Here's how the part is built. I have some questions about the finished solid (model axes, mm). A direction names the side the tool comes from. Round coordinates to 2 decimals unless told otherwise and drop trailing zeros. Loops run counter-clockwise (first coordinate to the right, second up) from the corner with the lowest first, then second, coordinate; pieces in that order, holes last. Notation, with made-up numbers: M -9.75,60 L 39.25,60 A17 ccw 39.25,90 Z; hole C 51.25,20.25 d4. An arc over 180 degrees is marked long. Use a Markdown table: item, result.
from build123d import *

# Parameters (mm, degrees)
SKETCH1_W                 = 101.6
SKETCH1_H                 = 48.26
BOSS_EXTRUDE1_DEPTH       = 38.1
SHELL1_T                  = -7.62
SKETCH4_W                 = 22.86
SKETCH4_H                 = 10.16
CUT_EXTRUDE1_DEPTH        = 38.1
SKETCH5_W                 = 33.02
SKETCH5_H                 = 7.62
CUT_EXTRUDE2_DEPTH        = 80.757617818
F_8_32_TAPPED_HOLE1_D     = 3.4544
F_8_32_TAPPED_HOLE1_DEPTH = 12.065
F_8_32_TAPPED_HOLE1_TIP   = 1.037806461


with BuildPart() as part:
    # Sketch1 → Boss-Extrude1 (new body)
    with BuildSketch(Plane(origin=(0, 0, 0), x_dir=(1, 0, 0), z_dir=(0, 1, 0))):
        Rectangle(SKETCH1_W, SKETCH1_H)
    extrude(amount=BOSS_EXTRUDE1_DEPTH)

    # Shell1
    shell1_openings = [part.faces().sort_by_distance(p)[0] for p in [
        (0, 38.1, 0),
    ]]
    offset(amount=SHELL1_T, openings=shell1_openings, kind=Kind.INTERSECTION)

    # Sketch4 → Cut-Extrude1 (cut)
    with BuildSketch(Plane.ZY.offset(50.8)):
        with Locations((0, 19.685)):
            Rectangle(SKETCH4_W, SKETCH4_H)
    extrude(amount=-CUT_EXTRUDE1_DEPTH, mode=Mode.SUBTRACT)

    # Sketch5 → Cut-Extrude2 (cut, through all)
    with BuildSketch(Plane(origin=(0, 0, -24.13), x_dir=(-1, 0, 0), z_dir=(0, 0, -1))):
        with Locations((-21.234297506, 19.685)):
            Rectangle(SKETCH5_W, SKETCH5_H)
    extrude(amount=-CUT_EXTRUDE2_DEPTH, mode=Mode.SUBTRACT)

    # #8-32 Tapped Hole1
    with Locations(Plane(origin=(0, 38.1, 0), x_dir=(1, 0, 0), z_dir=(0, 1, 0))):
        with Locations((46.99, -20.32), (26.67, 0), (46.99, 20.32), (6.35, -20.32), (6.35, 20.32)):
            Hole(F_8_32_TAPPED_HOLE1_D / 2, depth=F_8_32_TAPPED_HOLE1_DEPTH)
            with Locations((0, 0, -(F_8_32_TAPPED_HOLE1_DEPTH + F_8_32_TAPPED_HOLE1_TIP / 2))):  # 118° drill point
                Cone(0, F_8_32_TAPPED_HOLE1_D / 2, F_8_32_TAPPED_HOLE1_TIP, mode=Mode.SUBTRACT)


solid = part.part
1. Which directions (+Z, -Z, +X, -X, +Y, -Y) give clear straight access to the entire face, cutting with the end or side of a thin tool? Please do faces 1 (the face through (-47, 20, 11.43)), 2 (the face through (50.8, 19, 0)), 3 (the face through (-50.8, 10, 0)), 4 (the face through (5.421, 31.983, -21.776)), 5 (the face through (37.744, 20, 20)).
Answer sheet:
| item | result |
|---|---|
| face 1 | -X |
| face 2 | +Z, -Z, +X, +Y, -Y |
| face 3 | +Z, -Z, -X, +Y, -Y |
| face 4 | +Y |
| face 5 | +Z, -Z |
2. Imagine slicing it at D-D, the plane y = 34. Write out the boundary of the cut face in (x, z), then the cut area to 3 significant figures.
Answer sheet:
| item | result |
|---|---|
| outline | M -50.8,-24.13 L 50.8,-24.13 L 50.8,24.13 L -50.8,24.13 Z; hole M -43.18,-16.51 L 43.18,-16.51 L 43.18,16.51 L -43.18,16.51 Z; hole C 6.35,-20.32 d3.45; hole C 6.35,20.32 d3.45; hole C 46.99,-20.32 d3.45; hole C 46.99,20.32 d3.45 |
| area | 2,010 mm2 |
3. Imagine slicing it at A-A, the plane x = 9.5. Write out the boundary of the cut face in (y, z) (3 decimals), then the cut area to 3 significant figures.
Answer sheet:
| item | result |
|---|---|
| outline | M 0,-24.13 L 15.875,-24.13 L 15.875,-16.51 L 7.62,-16.51 L 7.62,16.51 L 15.875,16.51 L 15.875,24.13 L 0,24.13 Z; M 23.495,-24.13 L 38.1,-24.13 L 38.1,-16.51 L 23.495,-16.51 Z; M 23.495,16.51 L 38.1,16.51 L 38.1,24.13 L 23.495,24.13 Z |
| area | 716 mm2 |
4. Imagine slicing it at B-B, the plane y = 19.5. Write out the boundary of the cut face in (x, z).
Answer sheet:
| item | result |
|---|---|
| outline | M -50.8,-24.13 L 4.72,-24.13 L 4.72,-16.51 L -43.18,-16.51 L -43.18,-11.43 L -50.8,-11.43 Z; M -50.8,11.43 L -43.18,11.43 L -43.18,16.51 L 4.72,16.51 L 4.72,24.13 L -50.8,24.13 Z; M 37.74,-24.13 L 50.8,-24.13 L 50.8,24.13 L 37.74,24.13 L 37.74,16.51 L 43.18,16.51 L 43.18,-16.51 L 37.74,-16.51 Z |
5. We'd pull the mould along Y, two halves only. Please class faces 6 (the face through (-1, 19, 24.13)), 7 (the face through (47.151, 25.177, -20.573)), 8 (the face through (-47, 14.605, 0)): +Y half, -Y half, draft (parallel to the pull), parting line (faces both ways), or undercut.
Answer sheet:
| item | result |
|---|---|
| face 6 | draft |
| face 7 | +Y half |
| face 8 | undercut |
6. For pin 1 Ø1.5 at (x, z) = (-17.5, -4) entering from +Y, with a flat end and sliding along its axis, tell me the tip position at first contact or that it passes through.
Answer sheet:
| item | result |
|---|---|
| pin 1 | y = 7.62 |
7. Imagine slicing it at C-C, the plane z = 5. Write out the boundary of the cut face in (x, y) (3 decimals).
Answer sheet:
| item | result |
|---|---|
| outline | M -50.8,0 L 50.8,0 L 50.8,38.1 L 43.18,38.1 L 43.18,7.62 L -43.18,7.62 L -43.18,14.605 L -50.8,14.605 Z; M -50.8,24.765 L -43.18,24.765 L -43.18,38.1 L -50.8,38.1 Z |
8. I need wall thicknesses on probe 1 along X at (y, z) = (33.5, 20.32); probe 2 along Z at (x, y) = (6.35, 33.5); probe 3 along Z at (x, y) = (46.99, 31). Which ranges of each line are inside material? Lowest first, please. Write a range as from..to.
Answer sheet:
| item | result |
|---|---|
| probe 1 | -50.8..4.62, 8.08..45.26, 48.72..50.8 |
| probe 2 | -24.13..-22.05, -18.59..-16.51, 16.51..18.59, 22.05..24.13 |
| probe 3 | -24.13..-22.05, -18.59..18.59, 22.05..24.13 |
